Work out the finished part from the listing and answer in its coordinate system (mm). A direction names the side the tool comes from. Coordinates: 2 decimals unless noted, no trailing zeros. Write each loop counter-clockwise with the first axis right and the second up, starting at its lowest first coordinate (ties: lowest second). Pieces come first, ordered by that corner, then holes. Notation, with made-up numbers: (89.5, -10.75) - (138.5, -10.75) arc R34 cw to (138.5, 27.25) - close; hole circle Ø3 at (30.5, -22). An arc over 180 degrees is marked (long way). Answer as a JSON object with one key per item and string values. Group by question number.
Autodesk Inventor part; units mm, degrees
ref_plane "YZ Plane" through (0, 0, 0) normal (1, 0, 0) x (0, 1, 0)
ref_plane "XZ Plane" through (0, 0, 0) normal (0, 1, 0) x (-1, 0, 0)
ref_plane "XY Plane" through (0, 0, 0) normal (0, 0, 1) x (1, 0, 0)
sketch "Skizze1" plane through (0, 0, 0) normal (1, 0, 0) x (0, 1, 0)
  circle A0 centre (0, 0) radius 30
  dimension "d0" = 60
extrude "Extrusion1" add sketch "Skizze1" along normal blind 36
sketch "Skizze2" plane through (0, 0, 0) normal (0, 0, 1) x (1, 0, 0)
  line L0 (0, 30) -> (36, 30)
  line L1 (0, -30) -> (36, -30)
  line L2 (0, -30) -> (0, 30)
  line L3 (36, -30) -> (36, 30)
  line L4 (3, 30) -> (33, 30)
  line L5 (33, 30) -> (33, -30)
  line L6 (33, -30) -> (3, -30)
  line L7 (3, -30) -> (3, 30)
  point P0 (0, 0)
  dimension "d3" = 3
  dimension "d4" = 3
extrude "Extrusion2" cut sketch "Skizze2" along normal through all both and the other way through all contours L0 L5 L1 L7
sketch "Skizze3" plane through (3, 0, 0) normal (1, 0, 0) x (0, 0, -1)
  circle A0 centre (0, 0) radius 30
  circle A1 centre (0, 0) radius 8
  circle A2 centre (0, 0) radius 7
  point P0 (0, 0)
  dimension "d11" = 16
  dimension "d12" = 14
extrude "Extrusion3" add sketch "Skizze3" along normal blind 30 contours A1
sketch "Skizze4" plane through (36, 0, 0) normal (1, 0, 0) x (0, 0, -1)
  circle A0 centre (0, 0) radius 7
  circle A1 centre (0, 0) radius 7
  point P0 (0, 0)
extrude "Extrusion4" cut sketch "Skizze4" against normal through all
sketch "Skizze9" plane through (0, 0, 0) normal (0, 1, 0) x (-1, 0, 0)
  line L0 (0, 30) -> (-3, 30)
  line L1 (0, 30) -> (0, -30)
  circle A0 centre (-36, -179.9335) radius 209.9335
  line L2 (0, -208.9659) -> (0, 69.8277)
  line L3 (41.5282, 0) -> (-106.5298, 0)
  line L4 (-36, 30) -> (-36, -30)
  line L5 (-33, 30) -> (-36, 30)
  circle A1 centre (-36, -179.9335) radius 191.832
  circle A2 centre (-36, -179.9335) radius 168.168
  circle A3 centre (-36, -179.9335) radius 150.0665
  line L6 (-66, -32.8962) -> (-66, 27.8454)
  point P0 (0, 0)
  point P1 (-66, 9.5382)
  point P2 (-36, 11.8985)
  point P3 (-66, -14.463)
  point P4 (-36, -29.867)
  point P5 (-36, -11.7655)
  dimension "d25" = 300.133
  dimension "d21" = 36
  dimension "d22" = 419.867
  dimension "d23" = 383.664
  dimension "d24" = 336.336
  dimension "d26" = 30
extrude "Extrusion6" add sketch "Skizze9" along normal mid plane 10.2 contours L4 A1 L6 A0 | L4 A3 L6 A2
sketch "Skizze10" plane through (0, 0, 0) normal (0, 0, 1) x (1, 0, 0)
  line L0 (36, 5.1) -> (36, 5.1)
  line L1 (36, 2.8218) -> (36, 5.1)
  line L2 (36, -2.8218) -> (36, 2.8218)
  line L3 (36, -5.1) -> (36, -2.8218)
  line L4 (36, -5.1) -> (36, -5.1)
  line L5 (36, 0) -> (36, -5.1)
  line L6 (36, 5.1) -> (36, 0)
  line L7 (33, -30) -> (33, 30)
  line L8 (36, -5.1) -> (36, 0)
  line L9 (36, 0) -> (36, 5.1)
  line L10 (66, -5.1) -> (66, 5.1)
  line L11 (36, 2.1) -> (66, 2.1)
  line L12 (66, 2.1) -> (66, -2.1)
  line L13 (66, -2.1) -> (36, -2.1)
  line L14 (36, -2.1) -> (36, 2.1)
  line L15 (36, -5.1) -> (66, -5.1)
  line L16 (36, 5.1) -> (66, 5.1)
  point P0 (0, 0)
  point P1 (36, -3.1)
  point P2 (36, 3.1)
  dimension "d29" = 3
  dimension "d45" = 3
extrude "Extrusion8" cut sketch "Skizze10" along normal through all both and the other way through all contours L11 L10 L13 L2
sketch "Skizze11" plane through (0, 5.1, 0) normal (0, 1, 0) x (1, 0, 0)
  circle A0 centre (36, 179.9335) radius 159.1175
  line L0 (-245.2362, 0) -> (317.2362, 0)
  line L1 (0, 462.9798) -> (0, -112.1633)
  line L2 (36, -29.5633) -> (36, 29.5633)
  arc A1 (36, 29.867) -> (66, 32.8962) centre (36, 179.9335) ccw
  circle A2 centre (36, 179.9335) radius 200.883
  point P0 (0, 0)
  point P1 (51, 21.5246)
  point P2 (51, -20.3887)
  dimension "d34" = 318.235
  dimension "d36" = 401.766
  dimension "d35" = 15
  dimension "d37" = 15
hole "Bohrung1" at (51, 5.1, -21.5246) at (51, 5.1, 20.3887) direction (0, -1, 0) diameter 4 depth 50 tip angle 118
ref_plane "Arbeitsebene1" through (18, 0, 0) normal (1, 0, 0) x (0, 0, -1)
mirror "Spiegeln1" about plane through (18, 0, 0) normal (1, 0, 0) of "Extrusion6", "Bohrung1", "Extrusion8"
properties part number "Verbindungsstück"
Q1. Section A-A on z = 0 is taken. Determine the outline of the cut face in (x, y), plus the area to 3 significant figures.
Q2. Consider L1, parallel to Y at x = -23, z = -21; L2, parallel to X at y = -21, z = -4.5; L3, parallel to Z at x = -15, y = -3. Determine where each line is inside the solid, lowest interval first. Write a range as from..to.
Q3. A tool of negligible diameter and unlimited length cuts with its end or side. For faces 1 (the face through (51.27, 3.58, -12.46)), 2 (the face through (-15, 5.1, 18)), 3 (the face through (51.287, -3.621, -30.648)), from which of +Z, -Z, +X, -X, +Y, -Y can it reach the whole face along a straight path? Write none if from no direction.
Q4. Section C-C on x = 51 is taken. Count the separate pieces of the cut face and the enclosed holes in it, plus the area to 3 significant figures.
Q5. For a pull along Y with two mould halves and no side action, classify faces 4 (the face through (-15, -2.1, 17)), 5 (the face through (51, -5.1, 18)), 6 (the face through (52.774, -3.621, -20.602)) as +Y half, -Y half, draft (parallel to the pull), parting line (faces both ways), or undercut.
Q6. Section D-D on y = -12 is taken. Determine the outline of the cut face in (x, z).
Q7. Flat-ended cylindrical pins translate along their axes: pin 1 Ø18 at (y, z) = (-12.5, -3.5) entering from +X; pin 2 Ø5 at (x, z) = (48.5, -17) entering from -Y; pin 3 Ø10 at (y, z) = (20.5, 21.5) entering from -X. Find the tip coordinate at first contact, or state that the pin passes through.
Numbers:
{
 "1": {"outline": "(0, -30) - (3, -30) - (3, -8) - (33, -8) - (33, -30) - (36, -30) - (36, -7) - (0, -7) - close; (0, 7) - (36, 7) - (36, 30) - (33, 30) - (33, 8) - (3, 8) - (3, 30) - (0, 30) - close", "area": "336 mm²"},
 "2": {"L1": "y = -5.1..-2.1, 2.1..5.1", "L2": "x = 0..3, 33..36", "L3": "z = -30.62..-23.52, -19.52..-12.44, 11.31..18.39, 22.39..29.46"},
 "3": {"face 1": "+X, +Y, -Y", "face 2": "+Z, -Z, -X, +Y", "face 3": "-Z, +Y, -Y"},
 "4": {"separate pieces": "8", "enclosed holes": "0", "area": "170 mm²"},
 "5": {"face 4": "undercut", "face 5": "-Y half", "face 6": "draft"},
 "6": {"outline": "(0, -27.5) - (3, -27.5) - (3, 27.5) - (0, 27.5) - close; (33, -27.5) - (36, -27.5) - (36, 27.5) - (33, 27.5) - close"},
 "7": {"pin 1": "stops at x = 36", "pin 2": "stops at y = -5.1", "pin 3": "stops at x = 0"}
}
